Build history of the part. All positions in model axes, mm. A direction names the side the tool comes from. Round coordinates to 2 decimals unless told otherwise and drop trailing zeros. Loops run counter-clockwise (first coordinate to the right, second up) from the corner with the lowest first, then second, coordinate; pieces in that order, holes last.
from build123d import *

# Parameters (mm, degrees)
EXTRUDE_1_DEPTH     = 5
SKETCH_5_W          = 40
SKETCH_5_H          = 40
CUT_EXTRUDE_1_DEPTH = 2
SKETCH_7_R          = 2.5
CUT_EXTRUDE_2_DEPTH = 1.6
SKETCH_8_R          = 2.6
CUT_EXTRUDE_3_DEPTH = 1.6
SKETCH_9_R          = 5.1
CUT_EXTRUDE_4_DEPTH = 1.6


with BuildPart() as part:
    # 草图4 → 凸台-拉伸1 (new body)
    with BuildSketch(Plane(origin=(0, 0, 0), x_dir=(1, 0, 0), z_dir=(0, 1, 0))):
        Polygon((-85, 0), (0, 0), (85, 0), (85, 64), (-85, 64), align=None)
        Polygon((85, 0), (0, 0), (-85, 0), (-85, -64), (85, -64), align=None)
    extrude(amount=EXTRUDE_1_DEPTH)

    # 草图5 → 切除-拉伸1 (cut)
    with BuildSketch(Plane(origin=(0, 5, 0), x_dir=(1, 0, 0), z_dir=(0, 1, 0))):
        with Locations((-21, 42)):
            Rectangle(SKETCH_5_W, SKETCH_5_H)
        with Locations((-63, 42)):
            Rectangle(SKETCH_5_W, SKETCH_5_H)
        with Locations((21, 42)):
            Rectangle(SKETCH_5_W, SKETCH_5_H)
        with Locations((63, 42)):
            Rectangle(SKETCH_5_W, SKETCH_5_H)
        with Locations((-21, 0)):
            Rectangle(SKETCH_5_W, SKETCH_5_H)
        with Locations((21, 0)):
            Rectangle(SKETCH_5_W, SKETCH_5_H)
        with Locations((63, 0)):
            Rectangle(SKETCH_5_W, SKETCH_5_H)
        with Locations((-21, -42)):
            Rectangle(SKETCH_5_W, SKETCH_5_H)
        with Locations((21, -42)):
            Rectangle(SKETCH_5_W, SKETCH_5_H)
        with Locations((63, -42)):
            Rectangle(SKETCH_5_W, SKETCH_5_H)
        with Locations((-63, 0)):
            Rectangle(SKETCH_5_W, SKETCH_5_H)
        with Locations((-63, -42)):
            Rectangle(SKETCH_5_W, SKETCH_5_H)
    extrude(amount=-CUT_EXTRUDE_1_DEPTH, mode=Mode.SUBTRACT)

    # 草图7 → 切除-拉伸2 (cut)
    with BuildSketch(Plane.XZ):
        with Locations(Location((-50, 40, 0), (0, 0, 270))):
            Circle(SKETCH_7_R)
        with Locations(Location((50, 40, 0), (0, 0, 270))):
            Circle(SKETCH_7_R)
        with Locations(Location((50, -40, 0), (0, 0, 270))):
            Circle(SKETCH_7_R)
        with Locations(Location((-50, -40, 0), (0, 0, 270))):
            Circle(SKETCH_7_R)
    extrude(amount=-CUT_EXTRUDE_2_DEPTH, mode=Mode.SUBTRACT)

    # 草图8 → 切除-拉伸3 (cut)
    with BuildSketch(Plane.XZ):
        with Locations(Location((-50, 40, 0), (0, 0, 270))):
            Circle(SKETCH_8_R)
        with Locations(Location((50, 40, 0), (0, 0, 270))):
            Circle(SKETCH_8_R)
        with Locations(Location((50, -40, 0), (0, 0, 270))):
            Circle(SKETCH_8_R)
        with Locations(Location((-50, -40, 0), (0, 0, 270))):
            Circle(SKETCH_8_R)
    extrude(amount=-CUT_EXTRUDE_3_DEPTH, mode=Mode.SUBTRACT)

    # 草图9 → 切除-拉伸4 (cut)
    with BuildSketch(Plane.XZ):
        with Locations(Location((-50, 40, 0), (0, 0, 270))):
            Circle(SKETCH_9_R)
        with Locations(Location((50, 40, 0), (0, 0, 270))):
            Circle(SKETCH_9_R)
        with Locations(Location((50, -40, 0), (0, 0, 270))):
            Circle(SKETCH_9_R)
        with Locations(Location((-50, -40, 0), (0, 0, 270))):
            Circle(SKETCH_9_R)
    extrude(amount=-CUT_EXTRUDE_4_DEPTH, mode=Mode.SUBTRACT)


solid = part.part
(1) Slice it at B-B on z = -6. List the corners of the cut face in (x, y).
Responses:
outline: (-85, 0) - (85, 0) - (85, 5) - (83, 5) - (83, 3) - (43, 3) - (43, 5) - (41, 5) - (41, 3) - (1, 3) - (1, 5) - (-1, 5) - (-1, 3) - (-41, 3) - (-41, 5) - (-43, 5) - (-43, 3) - (-83, 3) - (-83, 5) - (-85, 5) - close
(2) Pin check, flat tip, straight feed: P1, Ø12, axis at x = -28.5, z = -50.5, coming from the +Y side. Stop position of the tip, or through.
Responses:
P1: stops at y = 3
(3) Pull direction X, two halves, no side cores. Call faces 1 (the face through (85, 2, 1)), 2 (the face through (-1, 2, 64)), 3 (the face through (-63, 3, 42)): +X half, -X half, draft (parallel to the pull), parting line (faces both ways), or undercut.
Responses:
face 1: +X half
face 2: draft
face 3: undercut
(4) Slice it at C-C on y = 3.9. Count the separate pieces of the cut face and the enclosed holes in it, plus the area to 3 significant figures.
Responses:
separate pieces: 1
enclosed holes: 12
area: 2,560 mm2
(5) Probe line 1 (X direction, y = 0.7, z = -40); line 2 (X direction, y = 3.85, z = 5); line 3 (Y direction, x = 55.5, z = -29.5). List the from-to ranges inside material, lowest first.
Responses:
line 1: x = -85 to -55.1, -44.9 to 44.9, 55.1 to 85
line 2: x = -85 to -83, -43 to -41, -1 to 1, 41 to 43, 83 to 85
line 3: y = 0 to 3
(6) Which spindle directions (+Z, -Z, +X, -X, +Y, -Y) get a long thin tool onto all of the face, cutting with end or side? Do faces 4 (the face through (-1, 0, -1)), 5 (the face through (50, 1.6, 40)), 6 (the face through (-21, 3, 0)). Say none if no direction does.
Responses:
face 4: +Z, -Z, +X, -X, -Y
face 5: -Y
face 6: +Y
(7) Slice it at D-D on z = -40. List the corners of the cut face in (x, y), plus the area to 3 significant figures.
Responses:
outline: (-85, 0) - (-55.1, 0) - (-55.1, 1.6) - (-44.9, 1.6) - (-44.9, 0) - (44.9, 0) - (44.9, 1.6) - (55.1, 1.6) - (55.1, 0) - (85, 0) - (85, 5) - (83, 5) - (83, 3) - (43, 3) - (43, 5) - (41, 5) - (41, 3) - (1, 3) - (1, 5) - (-1, 5) - (-1, 3) - (-41, 3) - (-41, 5) - (-43, 5) - (-43, 3) - (-83, 3) - (-83, 5) - (-85, 5) - close
area: 497 mm2
(8) Slice it at A-A on x = 50. List the corners of the cut face in (y, z).
Responses:
outline: (0, -64) - (5, -64) - (5, -62) - (3, -62) - (3, -22) - (5, -22) - (5, -20) - (3, -20) - (3, 20) - (5, 20) - (5, 22) - (3, 22) - (3, 62) - (5, 62) - (5, 64) - (0, 64) - (0, 45.1) - (1.6, 45.1) - (1.6, 34.9) - (0, 34.9) - (0, -34.9) - (1.6, -34.9) - (1.6, -45.1) - (0, -45.1) - close
